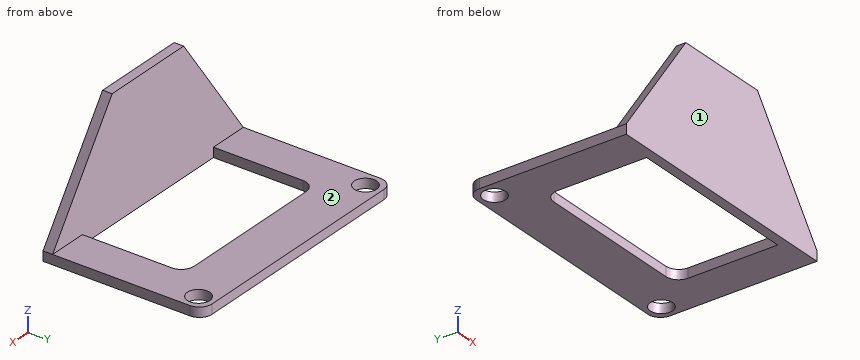
```python
from build123d import *

# Parameters (mm, degrees)
SKETCH_1_R      = 3.5
EXTRUDE_1_DEPTH = 3
FILLET_1_R      = 4
FILLET_2_R      = 4
FILLET_3_R      = 4
FILLET_4_R      = 4
EXTRUDE_2_DEPTH = 3


with BuildPart() as part:
    # 草图1 → 凸台-拉伸1 (new body)
    with BuildSketch(Plane.XY):
        Polygon((0, 0), (80, 0), (80, -50), (67.5, -50), (67.5, -15), (12.5, -15), (12.5, -50), (0, -50), align=None)
        with Locations((5, -5)):
            Circle(SKETCH_1_R, mode=Mode.SUBTRACT)
        with Locations((75, -5)):
            Circle(SKETCH_1_R, mode=Mode.SUBTRACT)
    extrude(amount=EXTRUDE_1_DEPTH)

    # 圆角1
    fillet_1_edges = [part.edges().sort_by_distance(p)[0] for p in [
        (0, 0, 1.5),
    ]]
    fillet(fillet_1_edges, radius=FILLET_1_R)

    # 圆角2
    fillet_2_edges = [part.edges().sort_by_distance(p)[0] for p in [
        (80, 0, 1.5),
    ]]
    fillet(fillet_2_edges, radius=FILLET_2_R)

    # 圆角3
    fillet_3_edges = [part.edges().sort_by_distance(p)[0] for p in [
        (12.5, -15, 1.5),
    ]]
    fillet(fillet_3_edges, radius=FILLET_3_R)

    # 圆角4
    fillet_4_edges = [part.edges().sort_by_distance(p)[0] for p in [
        (67.5, -15, 1.5),
    ]]
    fillet(fillet_4_edges, radius=FILLET_4_R)

    # 草图2 → 凸台-拉伸2 (add)
    with BuildSketch(Plane.XZ.offset(50)):
        Polygon((0, 3), (25, 38), (55, 38), (80, 3), (80, 0), (0, 0), align=None)
    extrude(amount=-EXTRUDE_2_DEPTH)


solid = part.part
```
Verification items for the finished model (mm, model axes). Face numbers are marked on the shaded views. A direction names the side the tool comes from. Coordinates: 2 decimals unless noted, no trailing zeros. Loops run counter-clockwise (first coordinate to the right, second up) from the corner with the lowest first, then second, coordinate; pieces in that order, holes last. Notation, with made-up numbers: (-11.75, 48.5) - (-1.75, 48.5) arc R29 cw to (-1.75, 72.5) - close; hole circle Ø1 at (73, 66.5). An arc over 180 degrees is marked (long way). Answer as a JSON object with one key per item and string values.
(1) Scan lines: line 1 along Y through (x, z) = (5, 2); line 2 along Y through (x, z) = (16, 14.5); line 3 along Z through (x, y) = (60.5, -14). Record each from-to range of solid material in increasing order.
Response:
{"line 1": "y = -50 to -8.5, -1.5 to 0", "line 2": "y = -50 to -47", "line 3": "z = 0 to 3"}
(2) Cross-section at A-A, the plane x = 39. Record the boundary of the cut face in (y, z).
Response:
{"outline": "(-50, 0) - (-47, 0) - (-47, 38) - (-50, 38) - close; (-15, 0) - (0, 0) - (0, 3) - (-15, 3) - close"}
(3) Go/stop test with flat-tipped pins: pin 1 Ø12 at (x, y) = (24.5, -18.5) entering from +Z; pin 2 Ø4 at (x, y) = (75, -5) entering from -Z; pin 3 Ø4 at (x, z) = (25.5, 6) entering from +Y. Record where each tip stops, or that it passes through.
Response:
{"pin 1": "stops at z = 3", "pin 2": "passes through", "pin 3": "stops at y = -47"}
(4) Cross-section at B-B, the plane y = -5. Record the boundary of the cut face in (x, z), then the cut area to 3 significant figures.
Response:
{"outline": "(0, 0) - (1.5, 0) - (1.5, 3) - (0, 3) - close; (8.5, 0) - (71.5, 0) - (71.5, 3) - (8.5, 3) - close; (78.5, 0) - (80, 0) - (80, 3) - (78.5, 3) - close", "area": "198 mm²"}
(5) Access from +Z, -Z, +X, -X, +Y, -Y to the whole of each face (thin tool, end or side, straight path). Record for the marked faces 1 and 2.
Response:
{"face 1": "+Z, -Z, +X, -X, -Y", "face 2": "+Z, +X, -X, +Y"}
(6) Cross-section at C-C, the plane y = -23. Record the boundary of the cut face in (x, z), then the cut area to 3 significant figures.
Response:
{"outline": "(0, 0) - (12.5, 0) - (12.5, 3) - (0, 3) - close; (67.5, 0) - (80, 0) - (80, 3) - (67.5, 3) - close", "area": "75.0 mm²"}
(7) Cross-section at D-D, the plane x = 5. Record the boundary of the cut face in (y, z), then the cut area to 3 significant figures.
Response:
{"outline": "(-50, 0) - (-8.5, 0) - (-8.5, 3) - (-47, 3) - (-47, 10) - (-50, 10) - close; (-1.5, 0) - (0, 0) - (0, 3) - (-1.5, 3) - close", "area": "150 mm²"}
